Here's how the part is built. I have some questions about the finished solid (model axes, mm). A direction names the side the tool comes from. Coordinates: 2 decimals unless noted, no trailing zeros. Write each loop counter-clockwise with the first axis right and the second up, starting at its lowest first coordinate (ties: lowest second). Pieces come first, ordered by that corner, then holes. Notation, with made-up numbers: (38.5, 50) -> (56.5, 50) arc R19 cw to (56.5, 72) -> close; hole circle Ø10 at (89, -7.5). An arc over 180 degrees is marked (long way). Answer in a Markdown table with one row per item. Add a question column.
from build123d import *

# Parameters (mm, degrees)
SKETCH1_R                = 9.525
BOSS_EXTRUDE1_DEPTH      = 19.05
BOSS_EXTRUDE2_DEPTH      = 6.35
BOSS_EXTRUDE2_DEPTH_BACK = 25.4
SKETCH2_R                = 3.1623
CUT_EXTRUDE1_DEPTH       = 29.750847814
CUT_EXTRUDE1_DEPTH_BACK  = 29.750847814
SKETCH3_R                = 3.9751


with BuildPart() as part:
    # Sketch1 → Boss-Extrude1 (new body)
    with BuildSketch(Plane.XY):
        with Locations(Location((0, 0, 0), (0, 0, 180))):
            Circle(SKETCH1_R)
    extrude(amount=BOSS_EXTRUDE1_DEPTH)

    # Sketch2 → Boss-Extrude2 (add, two sides: drawn at the far end of the back side and taken through both)
    with BuildSketch(Plane.XY.offset(19.05).offset(-BOSS_EXTRUDE2_DEPTH_BACK)):
        Circle(SKETCH2_R)
    extrude(amount=BOSS_EXTRUDE2_DEPTH + BOSS_EXTRUDE2_DEPTH_BACK)

    # Sketch3 → Cut-Extrude1 (cut, two sides: drawn at the far end of the back side and taken through both)
    with BuildSketch(Plane(origin=(0, 0, 0), x_dir=(0, 0, -1), z_dir=(1, 0, 0)).offset(-CUT_EXTRUDE1_DEPTH_BACK)):
        with Locations((-9.525, 0)):
            Circle(SKETCH3_R)
    extrude(amount=CUT_EXTRUDE1_DEPTH + CUT_EXTRUDE1_DEPTH_BACK, mode=Mode.SUBTRACT)


solid = part.part
Q1. If we mould it in two halves opening along Y, with no side actions, what happens to faces 4 (the flat face through (0, 0, 25.4)), 5 (the cylindrical face through (-0.13, -1.52, 5.85)), 6 (the cylindrical face through (3, 1, -3))? For each: pulls with the +Y half, pulls with the -Y half, needs draft (parallel to the pull), parting line crosses it, or undercut.
Q2. Imagine slicing it at A-A on x = 0. Please give me the cut outline in (y, z) (3 decimals), plus the area to 3 significant figures.
Q3. Imagine slicing it at D-D on z = 8.5. Please give me the cut outline in (x, y) (3 decimals).
Q4. I'm going to push flat-ended pins straight in: P1, Ø2, axis at y = -6, z = 17.5, coming from the -X side; P2, Ø3, axis at y = -3, z = 4, coming from the +X side; P3, Ø6, axis at y = -7, z = 13, coming from the -X side; P4, Ø9.5, axis at x = 3, y = -4.5, coming from the -Z side. Where does each tip first touch, or does it pass through?
Q5. I need wall thicknesses on line 1 (Z direction, x = -0.25, y = 0); line 2 (Z direction, x = -8.5, y = 0); line 3 (Z direction, x = 1, y = 7). Which ranges of each line are inside material? Lowest first, please. Write a range as [from, to].
Q6. Imagine slicing it at C-C on z = 17. Please give me the cut outline in (x, y) (3 decimals), plus the area to 3 significant figures.
Q7. Imagine slicing it at B-B on y = 0. Please give me the cut outline in (x, z) (3 decimals).
Q8. For faces 1 (the flat face through (-4, 0, 19.05)), 2 (the flat face through (-4, 0, 0)), 3 (the cylindrical face through (7.559, 5.796, 9.392)), which set-ups out of +Z, -Z, +X, -X, +Y, -Y let a thin tool reach every point of the face, with its end or its side?
Result sheet:
| question | item | result |
|---|---|---|
| 1 | face 4 | needs draft |
| 1 | face 5 | undercut |
| 1 | face 6 | parting line crosses it |
| 2 | outline | (-9.525, 0) -> (-3.162, 0) -> (-3.162, -6.35) -> (3.162, -6.35) -> (3.162, 0) -> (9.525, 0) -> (9.525, 19.05) -> (3.162, 19.05) -> (3.162, 25.4) -> (-3.162, 25.4) -> (-3.162, 19.05) -> (-9.525, 19.05) -> close; hole circle Ø7.95 at (0, 9.525) |
| 2 | area | 394 mm^2 |
| 3 | outline | (-8.716, -3.841) arc R9.525 ccw to (8.716, -3.841) -> close; (-8.716, 3.841) -> (8.716, 3.841) arc R9.525 ccw to start |
| 4 | P1 | stops at x = -8.11 |
| 4 | P2 | stops at x = 9.41 |
| 4 | P3 | stops at x = -8.64 |
| 4 | P4 | stops at z = -6.35 |
| 5 | line 1 | z = [-6.35, 5.55], [13.5, 25.4] |
| 5 | line 2 | z = [0, 5.55], [13.5, 19.05] |
| 5 | line 3 | z = [0, 19.05] |
| 6 | outline | circle Ø19.05 at (0, 0) |
| 6 | area | 285 mm^2 |
| 7 | outline | (-9.525, 0) -> (-3.162, 0) -> (-3.162, -6.35) -> (3.162, -6.35) -> (3.162, 0) -> (9.525, 0) -> (9.525, 5.55) -> (-9.525, 5.55) -> close; (-9.525, 13.5) -> (9.525, 13.5) -> (9.525, 19.05) -> (3.162, 19.05) -> (3.162, 25.4) -> (-3.162, 25.4) -> (-3.162, 19.05) -> (-9.525, 19.05) -> close |
| 8 | face 1 | +Z |
| 8 | face 2 | -Z |
| 8 | face 3 | +Z, -Z |
